```python
from build123d import *

# Parameters (mm, degrees)
F0_W     = 50.8
F0_H     = 50.8
F1_DEPTH = 55.88
F2_R     = 12.7
F4_DEPTH = 7.62
F5_R     = 9.525
F6_DEPTH = 36.83


with BuildPart() as f1:
    # F0 (on Top) → F1 (new body)
    with BuildSketch(Plane.XY):
        Rectangle(F0_W, F0_H)
    extrude(amount=F1_DEPTH)

    # F2
    f2_edges = [f1.edges().sort_by_distance(p)[0] for p in [
        (-25.4, 25.4, 27.94),
        (25.4, -25.4, 27.94),
    ]]
    fillet(f2_edges, radius=F2_R)

    # F3 (on face) → F4 (cut)
    with BuildSketch(Plane.XY.offset(55.88)):
        with BuildLine():
            Line((25.4, 25.4), (15.24, 25.4))
            ThreePointArc((15.24, 25.4), (18.215795, 18.215795), (25.4, 15.24))
            Line((25.4, 15.24), (25.4, 25.4))
        make_face()
        with BuildLine():
            ThreePointArc((-15.24, -25.4), (-18.215795, -18.215795), (-25.4, -15.24))
            Line((-25.4, -15.24), (-25.4, -25.4))
            Line((-25.4, -25.4), (-15.24, -25.4))
        make_face()
    extrude(amount=-F4_DEPTH, mode=Mode.SUBTRACT)

    # F5 (on face) → F6 (join)
    with BuildSketch(Plane.XY.offset(55.88)):
        Circle(F5_R)
    extrude(amount=F6_DEPTH)


solid = f1.part
```
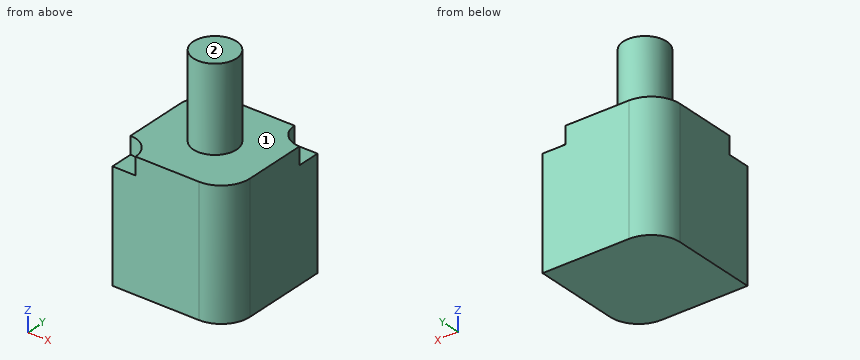
For this review, take the finished solid that the model builds, in its own axes (mm). Face numbers are marked on the shaded views. A direction names the side the tool comes from. Coordinates: 2 decimals unless noted, no trailing zeros. Order: outer loops, then holes, each group sorted by start corner. A loop starts at its lowest first (then second) coordinate and runs counter-clockwise, first axis right, second up. Notation, with made-up numbers: (25, -27.75) -> (36, -27.75) arc R14 ccw to (36, -23.75) -> close; hole circle Ø5 at (75, -2). An arc over 180 degrees is marked (long way). Use CSV: the item, a comma, the result in double quotes. Start each with the question number.
Item 1: We need section C-C, the plane z = 34. Give the boundary of the cut face in (x, y), then the cut area to 3 significant figures.
Item 2: Insertion check: pin 1 (10 mm diameter, centred on y = -7.5, z = 81.5, fed in from +X); pin 2 (12 mm diameter, centred on x = 20, y = 5, fed in from +Z); pin 3 (5 mm diameter, centred on x = 22, y = 20.5, fed in from +Z). Each pin has a flat end and moves straight along its axis. Give the tip position at first contact, or say it passes through.
Item 3: We need section D-D, the plane x = 16.5. Give the boundary of the cut face in (y, z).
Item 4: We need section A-A, the plane y = 0. Give the boundary of the cut face in (x, z) (3 decimals), then the cut area to 3 significant figures.
Item 5: For the marked faces 1 and 2, list the 3-axis set-ups (+Z, -Z, +X, -X, +Y, -Y) from which the entire face can be reached by the end or side of a thin tool; tool diameter is ignored.
Item 6: Wall thickness on probe 1 along Z at (x, y) = (7, 18); probe 2 along Y at (x, z) = (17, 28.5); probe 3 along X at (y, z) = (6.5, 87): over which ranges is each line inside the solid? List them lowest first.
Derived:
1,outline,"(-25.4, -25.4) -> (12.7, -25.4) arc R12.7 ccw to (25.4, -12.7) -> (25.4, 25.4) -> (-12.7, 25.4) arc R12.7 ccw to (-25.4, 12.7) -> close"
1,area,"2,510 mm^2"
2,pin 1,"stops at x = 9.19"
2,pin 2,"stops at z = 55.88"
2,pin 3,"stops at z = 48.26"
3,outline,"(-24.82, 0) -> (25.4, 0) -> (25.4, 48.26) -> (20.5, 48.26) -> (20.5, 55.88) -> (-24.82, 55.88) -> close"
4,outline,"(-25.4, 0) -> (25.4, 0) -> (25.4, 55.88) -> (9.525, 55.88) -> (9.525, 92.71) -> (-9.525, 92.71) -> (-9.525, 55.88) -> (-25.4, 55.88) -> close"
4,area,"3,540 mm^2"
5,face 1,"+Z"
5,face 2,"+Z, +X, -X, +Y, -Y"
6,probe 1,"z = 0 to 55.88"
6,probe 2,"y = -24.65 to 25.4"
6,probe 3,"x = -6.96 to 6.96"
